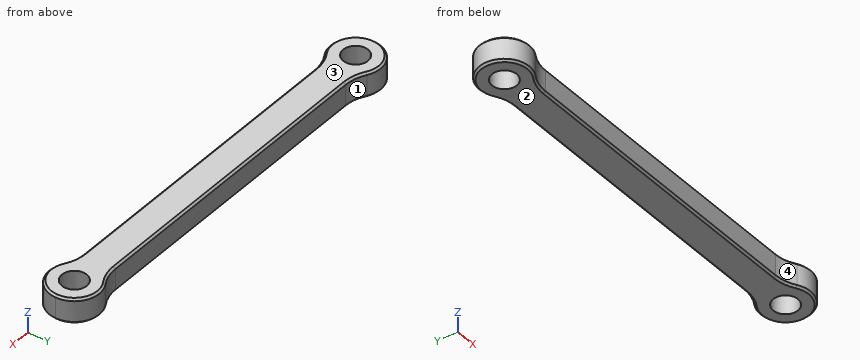
from build123d import *

# Parameters (mm, degrees)
SKETCH2_R           = 3.175
BOSS_EXTRUDE1_DEPTH = 6.35
FILLET1_R           = 10
CHAMFER1_SIZE       = 0.5


with BuildPart() as part:
    # Sketch2 → Boss-Extrude1 (new body)
    # profile 1 of 5: a face of its own
    with BuildSketch(Plane.XY):
        with BuildLine():
            Line((89.972015811, 4), (5.027984189, 4))
            ThreePointArc((5.027984189, 4), (6.065699606, 2.118469564), (6.425, 0))
            ThreePointArc((6.425, 0), (6.065699606, -2.118469564), (5.027984189, -4))
            Line((5.027984189, -4), (89.972015811, -4))
            ThreePointArc((89.972015811, -4), (88.575, 0), (89.972015811, 4))
        make_face()
    # profile 2 of 5: a face of its own
    with BuildSketch(Plane.XY):
        with BuildLine():
            Line((95, 4), (89.972015811, 4))
            ThreePointArc((89.972015811, 4), (88.575, 0), (89.972015811, -4))
            Line((89.972015811, -4), (95, -4))
            ThreePointArc((95, -4), (99, 0), (95, 4))
        make_face()
        with Locations((95, 0)):
            Circle(SKETCH2_R, mode=Mode.SUBTRACT)
    # profile 3 of 5: a face of its own
    with BuildSketch(Plane.XY):
        with BuildLine():
            ThreePointArc((101.425, 0), (97.118469564, 6.065699606), (89.972015811, 4))
            Line((89.972015811, 4), (95, 4))
            ThreePointArc((95, 4), (99, 0), (95, -4))
            Line((95, -4), (89.972015811, -4))
            ThreePointArc((89.972015811, -4), (97.118469564, -6.065699606), (101.425, 0))
        make_face()
    # profile 4 of 5: a face of its own
    with BuildSketch(Plane.XY):
        with BuildLine():
            Line((5.027984189, 4), (0, 4))
            ThreePointArc((0, 4), (-4, 0), (0, -4))
            Line((0, -4), (5.027984189, -4))
            ThreePointArc((5.027984189, -4), (6.065699606, -2.118469564), (6.425, 0))
            ThreePointArc((6.425, 0), (6.065699606, 2.118469564), (5.027984189, 4))
        make_face()
        Circle(SKETCH2_R, mode=Mode.SUBTRACT)
    # profile 5 of 5: a face of its own
    with BuildSketch(Plane.XY):
        with BuildLine():
            ThreePointArc((0, -4), (-4, 0), (0, 4))
            Line((0, 4), (5.027984189, 4))
            ThreePointArc((5.027984189, 4), (-6.425, 0), (5.027984189, -4))
            Line((5.027984189, -4), (0, -4))
        make_face()
    extrude(amount=BOSS_EXTRUDE1_DEPTH)

    # Fillet1
    fillet1_edges = [part.edges().sort_by_distance(p)[0] for p in [
        (89.972015811, 4, 3.175),
        (89.972015811, -4, 3.175),
        (5.027984189, -4, 3.175),
        (5.027984189, 4, 3.175),
    ]]
    fillet(fillet1_edges, radius=FILLET1_R)

    # Chamfer1
    chamfer1_edges = [part.edges().sort_by_distance(p)[0] for p in [
        (47.5, 4, 0),
        (47.5, 4, 6.35),
        (101.425, 0, 0),
        (101.425, 0, 6.35),
        (47.5, -4, 0),
        (47.5, -4, 6.35),
        (-6.425, 0, 0),
        (-6.425, 0, 6.35),
        (89.127426014, 4.376177452, 0),
        (89.127426014, 4.376177452, 6.35),
        (89.127426014, -4.376177452, 0),
        (89.127426014, -4.376177452, 6.35),
        (5.872573986, -4.376177452, 0),
        (5.872573986, -4.376177452, 6.35),
        (5.872573986, 4.376177452, 0),
        (5.872573986, 4.376177452, 6.35),
    ]]
    chamfer(chamfer1_edges, length=CHAMFER1_SIZE)


solid = part.part
Read the model definition and answer for the solid it produces. Units are mm, in the model's axes. Face numbers are marked on the shaded views. A direction names the side the tool comes from. Coordinates: 2 decimals unless noted, no trailing zeros. Write each loop counter-clockwise with the first axis right and the second up, starting at its lowest first coordinate (ties: lowest second). Pieces come first, ordered by that corner, then holes. Notation, with made-up numbers: M 14.5,-34 L 50.5,-34 A19 cw 50.5,-11 Z; hole C 81.5,-20.75 d11. An arc over 180 degrees is marked long. Use a Markdown table: item, result.
Q1. Each of these flat-tipped pins is pushed along its axis until it touches: pin 1 Ø2.5 at (x, z) = (56.5, 2) entering from -Y; pin 2 Ø1.5 at (x, z) = (71, 3.5) entering from +Y. Where does it stop, or does it pass through?
Answer block:
| item | result |
|---|---|
| pin 1 | stops at y = -4 |
| pin 2 | stops at y = 4 |
Q2. Which of the six approach directions +Z, -Z, +X, -X, +Y, -Y give full straight-line access (tool end or side, diameter ignored) to the marked faces 1 and 2?
Answer block:
| item | result |
|---|---|
| face 1 | +Z, -Z, +Y |
| face 2 | -Z, +X, -X, +Y, -Y |
Q3. The part is cut by section A-A, the plane z = 2.75. Write down the section's boundary in (x, y) (3 decimals).
Answer block:
| item | result |
|---|---|
| outline | M 3.36,-5.476 A10 cw 8.59,-4 L 86.41,-4 A10 cw 91.64,-5.476 A6.425 ccw long 91.64,5.476 A10 cw 86.41,4 L 8.59,4 A10 cw 3.36,5.476 A6.425 ccw long Z; hole C 0,0 d6.35; hole C 95,0 d6.35 |
Q4. The part is cut by section B-B, the plane x = 95. Write down the section's boundary in (y, z) (3 decimals), then the cut area to 3 significant figures.
Answer block:
| item | result |
|---|---|
| outline | M -6.425,0.5 L -5.925,0 L -3.175,0 L -3.175,6.35 L -5.925,6.35 L -6.425,5.85 Z; M 3.175,0 L 5.925,0 L 6.425,0.5 L 6.425,5.85 L 5.925,6.35 L 3.175,6.35 Z |
| area | 40.8 mm2 |
Q5. Determine the mould class of the marked faces 3 and 4 for opening direction X: released by +X, released by -X, zero draft, split by the parting line, or undercut.
Answer block:
| item | result |
|---|---|
| face 3 | zero draft |
| face 4 | undercut |
Q6. Straight lines are drawn through the part: L1, parallel to X at y = 0.25, z = 5.25; L2, parallel to Y at x = 0, z = 2.25 (3 decimals); L3, parallel to X at y = 1.5, z = 4.25. For each, find the intervals that lie inside material, in ascending order. Write a range as [from, to].
Answer block:
| item | result |
|---|---|
| L1 | x = [-6.42, -3.17], [3.17, 91.83], [98.17, 101.42] |
| L2 | y = [-6.425, -3.175], [3.175, 6.425] |
| L3 | x = [-6.25, -2.8], [2.8, 92.2], [97.8, 101.25] |
Q7. The part is cut by section C-C, the plane x = 20.5. Write down the section's boundary in (y, z), then the cut area to 3 significant figures.
Answer block:
| item | result |
|---|---|
| outline | M -4,0.5 L -3.5,0 L 3.5,0 L 4,0.5 L 4,5.85 L 3.5,6.35 L -3.5,6.35 L -4,5.85 Z |
| area | 50.3 mm2 |
